from build123d import *

# Parameters (mm, degrees)
F0_W     = 304.8
F0_H     = 203.2
F1_DEPTH = 203.2
F2_T     = -2.54
F4_D     = 8


with BuildPart() as f1:
    # F0 (on Right) → F1 (new body)
    with BuildSketch(Plane.YZ):
        with Locations((152.4, -101.6)):
            Rectangle(F0_W, F0_H)
    extrude(amount=F1_DEPTH)

    # F2
    f2_openings = [f1.faces().sort_by_distance(p)[0] for p in [
        (203.2, 152.4, -101.6),
    ]]
    offset(amount=F2_T, openings=f2_openings)

    # F4 (through all)
    with Locations(Plane.XZ):
        with Locations((152.4, -50.8), (152.4, -152.4)):
            Hole(F4_D / 2)


solid = f1.part
The listing builds one solid part. Answer for the finished solid, in the listing's coordinates (mm). A direction names the side the tool comes from. Give positions to 0.01 mm unless a question says otherwise; leave off trailing zeros. Loops run counter-clockwise (first coordinate to the right, second up) from the corner with the lowest first, then second, coordinate; pieces in that order, holes last. Notation, with made-up numbers: (54, 28) - (69, 28) arc R17 cw to (69, 58) - close; hole circle Ø6 at (13.25, -6). An arc over 180 degrees is marked (long way). Write each question's results on one line, items separated by ' | '.
1. Find section A-A, the plane x = 152.4. Write down the section's boundary in (y, z), then the cut area to 3 significant figures.
Resolved:
outline: (0, -203.2) - (304.8, -203.2) - (304.8, -156.4) - (302.26, -156.4) - (302.26, -200.66) - (2.54, -200.66) - (2.54, -156.4) - (0, -156.4) - close; (0, -148.4) - (2.54, -148.4) - (2.54, -54.8) - (0, -54.8) - close; (0, -46.8) - (2.54, -46.8) - (2.54, -2.54) - (302.26, -2.54) - (302.26, -46.8) - (304.8, -46.8) - (304.8, 0) - (0, 0) - close; (302.26, -148.4) - (304.8, -148.4) - (304.8, -54.8) - (302.26, -54.8) - close | area: 2,470 mm^2
2. Consider probe 1 along Z at (x, y) = (152.4, 303.5); probe 2 along Z at (x, y) = (167, 264.5); probe 3 along Y at (x, z) = (151, -169). Determine where each line is inside the solid, lowest interval first. Write a range as from..to.
Resolved:
probe 1: z = -203.2..-156.4, -148.4..-54.8, -46.8..0 | probe 2: z = -203.2..-200.66, -2.54..0 | probe 3: y = 0..2.54, 302.26..304.8
3. Find section D-D, the plane z = -21. Write down the section's boundary in (x, y).
Resolved:
outline: (0, 0) - (203.2, 0) - (203.2, 2.54) - (2.54, 2.54) - (2.54, 302.26) - (203.2, 302.26) - (203.2, 304.8) - (0, 304.8) - close
4. Which of the six approach directions +Z, -Z, +X, -X, +Y, -Y give full straight-line access (tool end or side, diameter ignored) to faces 5 (the face through (0, 150, -100)), 6 (the face through (101, 302.26, -103))?
Resolved:
face 5: +Z, -Z, -X, +Y, -Y | face 6: +X
5. For a pull along Z with two mould halves and no side action, classify faces 1 (the face through (2.54, 150, -100)), 2 (the face through (100, 0, -103)), 3 (the face through (100, 150, 0)), 4 (the face through (100, 150, -203.2)) as +Z half, -Z half, draft (parallel to the pull), parting line (faces both ways), or undercut.
Resolved:
face 1: undercut | face 2: draft | face 3: +Z half | face 4: -Z half
6. Find section B-B, the plane z = -152.4. Write down the section's boundary in (x, y).
Resolved:
outline: (0, 0) - (148.4, 0) - (148.4, 2.54) - (2.54, 2.54) - (2.54, 302.26) - (148.4, 302.26) - (148.4, 304.8) - (0, 304.8) - close; (156.4, 0) - (203.2, 0) - (203.2, 2.54) - (156.4, 2.54) - close; (156.4, 302.26) - (203.2, 302.26) - (203.2, 304.8) - (156.4, 304.8) - close
7. Flat-ended cylindrical pins translate along their axes: P1, Ø7, axis at x = 152.4, z = -152.4, coming from the -Y side; P2, Ø4, axis at y = 176.5, z = -153.5, coming from the +X side; P3, Ø4, axis at x = 138.5, z = -25, coming from the -Y side. Find the tip coordinate at first contact, or state that the pin passes through.
Resolved:
P1: passes through | P2: stops at x = 2.54 | P3: stops at y = 0
8. Find section C-C, the plane x = 64.5. Write down the section's boundary in (y, z), then the cut area to 3 significant figures.
Resolved:
outline: (0, -203.2) - (304.8, -203.2) - (304.8, 0) - (0, 0) - close; hole (2.54, -200.66) - (302.26, -200.66) - (302.26, -2.54) - (2.54, -2.54) - close | area: 2,550 mm^2
